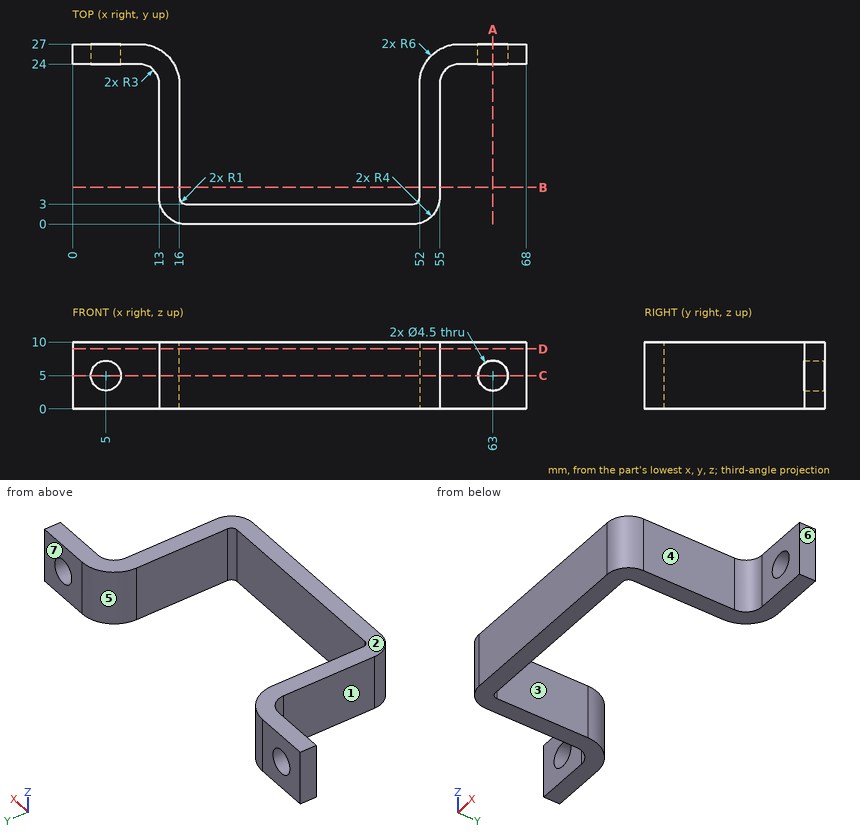
Geometry: see drawing. Coordinates: mm, zero at the bounding-box minimum. A direction names the side the tool comes from. Coordinates: 2 decimals unless noted, no trailing zeros. Loops run counter-clockwise (first coordinate to the right, second up) from the corner with the lowest first, then second, coordinate; pieces in that order, holes last. Notation, with made-up numbers: (11, 50) - (26, 50) arc R29 cw to (26, 83) - close; hole circle Ø8 at (43, 59.25). An arc over 180 degrees is marked (long way). Return JSON: item names as keys, results as strings.
Q1. Mould query, pull axis X, two halves, no side actions, for the marked faces 5, 6 and 7. Classes: released by +X, released by -X, zero draft, split by the parting line, or undercut.
Results:
{"face 5": "undercut", "face 6": "released by +X", "face 7": "zero draft"}
Q2. Section A-A, the plane x = 63. Return loops of the section in (y, z), plus the area to 3 significant figures.
Results:
{"outline": "(24, 0) - (27, 0) - (27, 2.75) - (24, 2.75) - close; (24, 7.25) - (27, 7.25) - (27, 10) - (24, 10) - close", "area": "16.5 mm2"}
Q3. Contact query for flat-ended pins moving along their axis: P1, Ø5, axis at y = 18.5, z = 3.5, coming from the -X side; P2, Ø5, axis at x = 5, z = 3, coming from the -Y side; P3, Ø3, axis at x = 28, z = 6, coming from the +Y side. Output: stop coordinate, or through.
Results:
{"P1": "x = 13", "P2": "y = 24", "P3": "y = 3"}
Q4. Material intervals for line 1 along X through (y, z) = (9, 1.75); line 2 along Z through (x, y) = (5, 24.95); line 3 along X through (y, z) = (25, 6.75), sorted ascending.
Results:
{"line 1": "13 to 16, 52 to 55", "line 2": "0 to 2.75, 7.25 to 10", "line 3": "0 to 3.59, 6.41 to 14.47, 53.53 to 61.59, 64.41 to 68"}
Q5. Section D-D, the plane z = 9. Return loops of the section in (x, y), plus the area to 3 significant figures.
Results:
{"outline": "(0, 24) - (10, 24) arc R3 cw to (13, 21) - (13, 4) arc R4 ccw to (17, 0) - (51, 0) arc R4 ccw to (55, 4) - (55, 21) arc R3 cw to (58, 24) - (68, 24) - (68, 27) - (58, 27) arc R6 ccw to (52, 21) - (52, 4) arc R1 cw to (51, 3) - (17, 3) arc R1 cw to (16, 4) - (16, 21) arc R6 ccw to (10, 27) - (0, 27) - close", "area": "330 mm2"}
Q6. Access query for the marked faces 1, 2, 3 and 4. Directions: +Z, -Z, +X, -X, +Y, -Y. A direction counts if a zero-diameter tool reaches every point of the face in a straight line with its end or side. Return the directions, or none.
Results:
{"face 1": "+Z, -Z, -X, -Y", "face 2": "+Z, +X, -X, +Y, -Y", "face 3": "+Z, -Z, +Y", "face 4": "+Z, -Z, +X, -Y"}
Q7. Section B-B, the plane y = 5.5. Return loops of the section in (x, z), plus the area to 3 significant figures.
Results:
{"outline": "(13, 0) - (16, 0) - (16, 10) - (13, 10) - close; (52, 0) - (55, 0) - (55, 10) - (52, 10) - close", "area": "60.0 mm2"}
Q8. Section C-C, the plane z = 5. Return loops of the section in (x, y), plus the area to 3 significant figures.
Results:
{"outline": "(0, 24) - (2.75, 24) - (2.75, 27) - (0, 27) - close; (7.25, 24) - (10, 24) arc R3 cw to (13, 21) - (13, 4) arc R4 ccw to (17, 0) - (51, 0) arc R4 ccw to (55, 4) - (55, 21) arc R3 cw to (58, 24) - (60.75, 24) - (60.75, 27) - (58, 27) arc R6 ccw to (52, 21) - (52, 4) arc R1 cw to (51, 3) - (17, 3) arc R1 cw to (16, 4) - (16, 21) arc R6 ccw to (10, 27) - (7.25, 27) - close; (65.25, 24) - (68, 24) - (68, 27) - (65.25, 27) - close", "area": "303 mm2"}
